from build123d import *

# Parameters (mm, degrees)
SKETCH2_W           = 20.475
SKETCH2_H           = 94.165655299
SKETCH2_R           = 1.725
SKETCH2_R_2         = 10
BOSS_EXTRUDE1_DEPTH = 3.175
SKETCH3_W           = 3.175
SKETCH3_H           = 40
SKETCH3_H_2         = 20
SKETCH3_W_2         = 40
SKETCH3_H_3         = 3.175
SKETCH3_W_3         = 20
CUT_EXTRUDE1_DEPTH  = 10
FILLET1_R           = 5


with BuildPart() as part:
    # Sketch2 → Boss-Extrude1 (new body)
    with BuildSketch(Plane(origin=(0, 0, 0), x_dir=(0, 0, -1), z_dir=(1, 0, 0))):
        Polygon((35, -119.825), (35, 117.5), (-35, 117.5), (-35, -117.5), (0, -117.5), (2.325, -119.825), align=None)
        with Locations((-15.2375, -49.067172351)):
            Rectangle(SKETCH2_W, SKETCH2_H, mode=Mode.SUBTRACT)
        with Locations((15.2375, -49.067172351)):
            Rectangle(SKETCH2_W, SKETCH2_H, mode=Mode.SUBTRACT)
        with Locations((5, 56.954767415)):
            Circle(SKETCH2_R, mode=Mode.SUBTRACT)
        with Locations((-5, 56.954767415)):
            Circle(SKETCH2_R, mode=Mode.SUBTRACT)
        with Locations((-5, 106.454767415)):
            Circle(SKETCH2_R, mode=Mode.SUBTRACT)
        with Locations((5, 106.454767415)):
            Circle(SKETCH2_R, mode=Mode.SUBTRACT)
        with Locations((0, 92.104767415)):
            Circle(SKETCH2_R_2, mode=Mode.SUBTRACT)
    extrude(amount=BOSS_EXTRUDE1_DEPTH)

    # Sketch3 → Cut-Extrude1 (cut)
    with BuildSketch(Plane.ZY):
        with Locations((-33.4125, 59.155293611)):
            Rectangle(SKETCH3_W, SKETCH3_H)
        with Locations((33.4125, 59.155293611)):
            Rectangle(SKETCH3_W, SKETCH3_H)
        with Locations((33.4125, 10)):
            Rectangle(SKETCH3_W, SKETCH3_H_2)
        with Locations((-33.4125, 10)):
            Rectangle(SKETCH3_W, SKETCH3_H_2)
        with Locations((-33.4125, -10)):
            Rectangle(SKETCH3_W, SKETCH3_H_2)
        with Locations((33.4125, -10)):
            Rectangle(SKETCH3_W, SKETCH3_H_2)
        with Locations((33.4125, -59.155293611)):
            Rectangle(SKETCH3_W, SKETCH3_H)
        with Locations((-33.4125, -59.155293611)):
            Rectangle(SKETCH3_W, SKETCH3_H)
        with Locations((0, 115.9125)):
            Rectangle(SKETCH3_W_2, SKETCH3_H_3)
        with Locations((17.5, -115.9125)):
            Rectangle(SKETCH3_W_3, SKETCH3_H_3)
    extrude(amount=-CUT_EXTRUDE1_DEPTH, mode=Mode.SUBTRACT)

    # Fillet1
    fillet1_edges = [part.edges().sort_by_distance(p)[0] for p in [
        (1.5875, -117.5, 35),
    ]]
    fillet(fillet1_edges, radius=FILLET1_R)


solid = part.part
Part model, mm, in its own coordinate system. Give positions to 0.01 mm unless a question says otherwise; leave off trailing zeros. Loops run counter-clockwise (first coordinate to the right, second up) from the corner with the lowest first, then second, coordinate; pieces in that order, holes last.
(1) Pin check, flat tips, straight feed: pin 1 (2 mm diameter, centred on y = 92.5, z = 26.5, fed in from -X); pin 2 (1.6 mm diameter, centred on x = 2, z = 34, fed in from -Y); pin 3 (1 mm diameter, centred on x = 1, y = -58.5, fed in from -Z) (3 decimals). Stop position of each tip, or through.
Return value:
pin 1: stops at x = 0
pin 2: stops at y = -116.34
pin 3: stops at z = -31.825
(2) Band-saw the part on B-B (y = 94.5). Write the cut outline in (x, z) (3 decimals), and give its area (3 significant figures).
Return value:
outline: (0, -35) - (3.175, -35) - (3.175, -9.709) - (0, -9.709) - close; (0, 9.709) - (3.175, 9.709) - (3.175, 35) - (0, 35) - close
area: 161 mm2
(3) Band-saw the part on D-D (x = 0.7). Count the separate pieces of the cut face and the enclosed holes in it, and give its area (3 significant figures).
Return value:
separate pieces: 1
enclosed holes: 7
area: 11,400 mm2
(4) Pull direction Y, two halves, no side cores. Call faces 1 (the cylindrical face through (1.57, 102.02, 1.3)), 2 (the flat face through (3.175, 27, 0)), 3 (the cylindrical face through (1.61, -116.07, 33.5)): pulls with the +Y half, pulls with the -Y half, needs draft (parallel to the pull), parting line crosses it, or undercut.
Return value:
face 1: undercut
face 2: needs draft
face 3: pulls with the -Y half
(5) Band-saw the part on C-C (y = -23.5). Write the cut outline in (x, z) (3 decimals).
Return value:
outline: (0, -35) - (3.175, -35) - (3.175, -25.475) - (0, -25.475) - close; (0, -5) - (3.175, -5) - (3.175, 5) - (0, 5) - close; (0, 25.475) - (3.175, 25.475) - (3.175, 35) - (0, 35) - close
(6) Band-saw the part on A-A (y = -52). Write the cut outline in (x, z) (3 decimals).
Return value:
outline: (0, -31.825) - (3.175, -31.825) - (3.175, -25.475) - (0, -25.475) - close; (0, -5) - (3.175, -5) - (3.175, 5) - (0, 5) - close; (0, 25.475) - (3.175, 25.475) - (3.175, 31.825) - (0, 31.825) - close
(7) Drill centre lines: line 1 along Z through (x, y) = (0.3, -31) (3 decimals); line 2 along Z through (x, y) = (3, -7) (3 decimals); line 3 along Y through (x, z) = (2.55, -21) (3 decimals). Where is each one in solid material? Low to high.
Return value:
line 1: z = -35 to -25.475, -5 to 5, 25.475 to 35
line 2: z = -31.825 to -25.475, -5 to 5, 25.475 to 31.825
line 3: y = -119.825 to -96.15, -1.984 to 117.5
